Study the drawing (mm; zero at the part's minimum x, y, z) and answer. A direction names the side the tool comes from. Coordinates: 2 decimals unless noted, no trailing zeros. Order: outer loops, then holes, each group sorted by start corner. A loop starts at its lowest first (then second) coordinate and runs counter-clockwise, first axis right, second up. Notation, with made-up numbers: M -7,-30.5 L 21,-30.5 A30 ccw 21,3.5 Z; hole C 49.5,-10 d8. An arc over 180 degrees is marked long. Put each result on its own line as item: value.
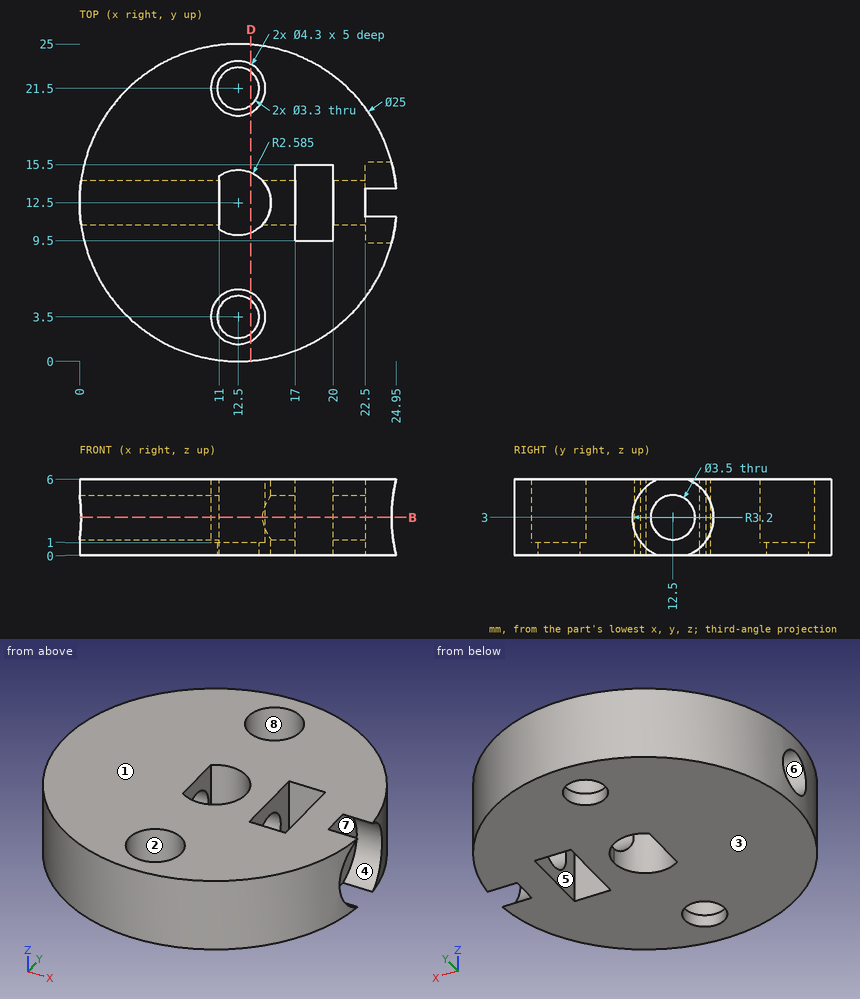
Q1. A tool of negligible diameter and unlimited length cuts with its end or side. For the marked faces 1, 2, 3, 4 and 5, from which of +Z, -Z, +X, -X, +Y, -Y can it reach the whole face along a straight path? Write none if from no direction.
Answers below:
face 1: +Z, +X, -X, +Y, -Y
face 2: +Z
face 3: -Z, +X, -X, +Y, -Y
face 4: +X
face 5: +Z, -Z
Q2. Find section D-D on x = 13.5. Write down the section's boundary in (y, z), plus the area to 3 significant figures.
Answers below:
outline: M 0.04,0 L 2.19,0 L 2.19,1 L 1.6,1 L 1.6,6 L 0.04,6 Z; M 4.81,0 L 10.12,0 L 10.12,6 L 5.4,6 L 5.4,1 L 4.81,1 Z; M 14.88,0 L 20.19,0 L 20.19,1 L 19.6,1 L 19.6,6 L 14.88,6 Z; M 22.81,0 L 24.96,0 L 24.96,6 L 23.4,6 L 23.4,1 L 22.81,1 Z
area: 77.6 mm^2
Q3. Given pin 1 (2 mm diameter, centred on x = 12.5, y = 3.5, fed in from -Z); pin 2 (1.5 mm diameter, centred on x = 21.5, z = 4.5, fed in from +Y); pin 3 (1 mm diameter, centred on x = 21.5, z = 2, fed in from -Y) (1 decimal); pin 4 (1.5 mm diameter, centred on x = 7.5, z = 2, fed in from -Y) (1 decimal), each flat-ended and moving along its own axis, determine where each tip first touches the part or whether it passes through.
Answers below:
pin 1: passes through
pin 2: stops at y = 21.89
pin 3: stops at y = 3.3
pin 4: stops at y = 0.7
Q4. Find section B-B on z = 3. Give the number of separate pieces and of enclosed holes in the cut face, plus the area to 3 significant figures.
Answers below:
separate pieces: 2
enclosed holes: 2
area: 356 mm^2
Q5. Consider line 1 along X through (y, z) = (14.5, 2); line 2 along Y through (x, z) = (11.25, 4.25); line 3 along Y through (x, z) = (13.25, 2.25) (1 decimal). Determine where each line is inside the solid, lowest interval first.
Answers below:
line 1: x = 0.16 to 11, 14.14 to 17, 20 to 22.5
line 2: y = 0.06 to 1.75, 5.25 to 10.24, 14.76 to 19.75, 23.25 to 24.94
line 3: y = 0 to 1.5, 5.5 to 10, 15 to 19.5, 23.5 to 25
Q6. For a pull along X with two mould halves and no side action, classify the marked faces 6, 7 and 8 as +X half, -X half, draft (parallel to the pull), parting line (faces both ways), or undercut.
Answers below:
face 6: draft
face 7: +X half
face 8: undercut
